from build123d import *

# Parameters (mm, degrees)
SKETCH2_R           = 19.05
BOSS_EXTRUDE1_DEPTH = 152.4
BOSS_EXTRUDE2_DEPTH = 12.7
SKETCH4_W           = 138.346275672
SKETCH4_H           = 79.731841005
BOSS_EXTRUDE3_DEPTH = 50.8
SKETCH5_W           = 63.5
SKETCH5_H           = 57.15
CUT_EXTRUDE1_DEPTH  = 132.116075905
CUT_EXTRUDE2_DEPTH  = 132.116075905
CUT_EXTRUDE3_DEPTH  = 124.514960069
SKETCH9_R           = 3.683
BOSS_EXTRUDE4_DEPTH = 25.4
CLEARANCECUT1_DEPTH = 109.569099969
CLEARANCECUT2_DEPTH = 12.954


with BuildPart() as part:
    # Sketch2 → Boss-Extrude1 (new body)
    with BuildSketch(Plane(origin=(0, 0, 0), x_dir=(1, 0, 0), z_dir=(0, 1, 0))):
        with Locations(Location((0, 0, 0), (0, 0, 90))):
            Circle(SKETCH2_R)
    extrude(amount=BOSS_EXTRUDE1_DEPTH)

    # Sketch3 → Boss-Extrude2 (add, symmetric)
    with BuildSketch(Plane.XY):
        Polygon((-427.750314484, -331.6732), (-409.789802242, -313.712687758), (-391.82929, -331.6732), align=None)
        Polygon((-6.028675512, 90.048438972), (-409.789802242, -313.712687758), (-391.82929, -331.6732), (11.93183673, 72.08792673), align=None)
    boss_extrude2 = extrude(amount=BOSS_EXTRUDE2_DEPTH, both=True)

    # Mirror1: Boss-Extrude2 across plane
    add(boss_extrude2.mirror(Plane(origin=(0, 0, 0), x_dir=(0, 0, 1), z_dir=(1, 0, 0))))


with BuildPart() as body_2:
    # Sketch4 → Boss-Extrude3 (new body)
    with BuildSketch(Plane.XY.offset(25.4)):
        with Locations((0, 59.259567455)):
            Rectangle(SKETCH4_W, SKETCH4_H)
    extrude(amount=-BOSS_EXTRUDE3_DEPTH)

    # Combine1: cut part
    add(part.part, mode=Mode.SUBTRACT)

    # Sketch5 → Cut-Extrude1 (cut, through all)
    with BuildSketch(Plane.XY.offset(25.4)):
        with Locations((0, 59.259567454)):
            Rectangle(SKETCH5_W, SKETCH5_H)
    extrude(amount=-CUT_EXTRUDE1_DEPTH, mode=Mode.SUBTRACT)

    # Sketch6 → Cut-Extrude2 (cut, through all)
    with BuildSketch(Plane.XY.offset(25.4)):
        Polygon((-69.173137836, 99.125487957), (-69.173137836, 44.864488891), (-40.730256121, 73.307370605), (-40.730256121, 99.125487957), align=None)
    cut_extrude2 = extrude(amount=-CUT_EXTRUDE2_DEPTH, mode=Mode.SUBTRACT)

    # Mirror2: Cut-Extrude2 across plane
    add(cut_extrude2.mirror(Plane(origin=(0, 0, 0), x_dir=(0, 0, 1), z_dir=(1, 0, 0))), mode=Mode.SUBTRACT)

    # Sketch8 → Cut-Extrude3 (cut, through all)
    with BuildSketch(Plane.XY):
        Polygon((69.173137836, 19.393646952), (69.173137836, 44.864488891), (40.730256121, 73.307370605), (40.730256121, 99.125487957), (-40.730256121, 99.125487957), (-40.730256121, 73.307370605), (-69.173137836, 44.864488891), (-69.173137836, 19.393646952), align=None)
    extrude(amount=-CUT_EXTRUDE3_DEPTH, mode=Mode.SUBTRACT)

    # Sketch9 → Boss-Extrude4 (add)
    with BuildSketch(Plane(origin=(0, 0, 0), x_dir=(-1, 0, 0), z_dir=(0, 0, -1))):
        with BuildLine():
            Line((-48.773997692, 65.263629035), (-39.369751391, 74.667875336))
            ThreePointArc((-39.369751391, 74.667875336), (-50.088798441, 81.199961636), (-52.36610014, 68.855731483))
            Line((-52.36610014, 68.855731483), (-48.773997692, 65.263629035))
        make_face()
        with Locations((-46.977946468, 74.243885156)):
            Circle(SKETCH9_R, mode=Mode.SUBTRACT)
    boss_extrude4 = extrude(amount=-BOSS_EXTRUDE4_DEPTH)

    # Mirror3: Boss-Extrude4 across plane
    add(boss_extrude4.mirror(Plane(origin=(0, 0, 0), x_dir=(0, 0, 1), z_dir=(1, 0, 0))))

    # Sketch10 → ClearanceCut1 (cut, through all)
    with BuildSketch(Plane.XZ.offset(-19.393646952)):
        with BuildLine():
            Line((-19.05, 0), (-19.304, 0))
            ThreePointArc((-19.304, 0), (0, 19.304), (19.304, 0))
            Line((19.304, 0), (19.05, 0))
            ThreePointArc((19.05, 0), (0, 19.05), (-19.05, 0))
        make_face()
    extrude(amount=-CLEARANCECUT1_DEPTH, mode=Mode.SUBTRACT)

    # Sketch11 → ClearanceCut2 (cut)
    with BuildSketch(Plane(origin=(0, 0, 0), x_dir=(-1, 0, 0), z_dir=(0, 0, -1))):
        Polygon((-69.173137836, 27.263186893), (-29.112312301, 67.324012428), (-29.112312301, 30.684567454), (-40.403232803, 19.393646952), (-69.173137836, 19.393646952), align=None)
    clearancecut2 = extrude(amount=-CLEARANCECUT2_DEPTH, mode=Mode.SUBTRACT)

    # Mirror4: ClearanceCut2 across plane
    add(clearancecut2.mirror(Plane(origin=(0, 0, 0), x_dir=(0, 0, 1), z_dir=(1, 0, 0))), mode=Mode.SUBTRACT)


solid = body_2.part
Build history of the part. All positions in model axes, mm. A direction names the side the tool comes from. Coordinates: 2 decimals unless noted, no trailing zeros. Order: outer loops, then holes, each group sorted by start corner. A loop starts at its lowest first (then second) coordinate and runs counter-clockwise, first axis right, second up. Notation, with made-up numbers: (-28.5, 7) - (-16.5, 7) arc R27 ccw to (-16.5, 42) - close; hole circle Ø11 at (70.25, 23). An arc over 180 degrees is marked (long way). Put each result on its own line as item: value.
1. Tool access for faces 4 (the face through (49, 32, 12.954)), 5 (the face through (59.12, 54.92, 12.88)), 6 (the face through (-59.12, 54.92, 12.88)), 7 (the face through (0, 30.685, 21)), 8 (the face through (69.173, 35, 13)): list every direction of +Z, -Z, +X, -X, +Y, -Y with a clear straight run to the whole face (end or side of a thin tool).
Answer sheet:
face 4: -Z
face 5: +Z, -Z, +X
face 6: +Z, -Z, -X
face 7: +Z, -Z
face 8: +Z, -Z, +X, +Y, -Y
2. Probe line 1 along X through (y, z) = (73, 11); line 2 along X through (y, z) = (71.5, 21.25); line 3 along Y through (x, z) = (3.5, 19.25). List the from-to ranges inside material, lowest first. Write a range as [from, to].
Answer sheet:
line 1: x = [-54.5, -50.44], [-43.51, -31.75], [31.75, 43.51], [50.44, 54.5]
line 2: x = [-54.09, -49.43], [-44.52, -31.75], [31.75, 44.52], [49.43, 54.09]
line 3: y = [19.39, 30.68], [87.83, 99.13]
3. Saw through at C-C (y = 53). Write the cut outline in (x, z).
Answer sheet:
outline: (-61.04, 0) - (-43.44, 0) - (-43.44, 12.95) - (-31.75, 12.95) - (-31.75, 25.4) - (-61.04, 25.4) - close; (31.75, 12.95) - (43.44, 12.95) - (43.44, 0) - (61.04, 0) - (61.04, 25.4) - (31.75, 25.4) - close
4. Saw through at D-D (x = 0). Write the cut outline in (y, z).
Answer sheet:
outline: (19.39, 19.3) - (30.68, 19.3) - (30.68, 25.4) - (19.39, 25.4) - close; (87.83, 19.3) - (99.13, 19.3) - (99.13, 25.4) - (87.83, 25.4) - close
5. Drop flat-ended pins along their axis: P1, Ø2, axis at x = 31, y = 32.5, coming from the -Z side; P2, Ø5, axis at y = 50, z = 21, coming from the -X side; P3, Ø2, axis at y = 54.5, z = 17, coming from the -X side. Give the stop position or say it passes through.
Answer sheet:
P1: stops at z = 12.95
P2: stops at x = -66.54
P3: stops at x = -60.54
6. Saw through at A-A (x = 27.5). Write the cut outline in (y, z), and give its area (3 significant figures).
Answer sheet:
outline: (19.39, 0) - (30.68, 0) - (30.68, 25.4) - (19.39, 25.4) - close; (87.83, 0) - (99.13, 0) - (99.13, 25.4) - (87.83, 25.4) - close
area: 574 mm^2
7. Saw through at B-B (z = 2). Give the number of separate pieces and of enclosed holes in the cut face, and give its area (3 significant figures).
Answer sheet:
separate pieces: 4
enclosed holes: 2
area: 2,570 mm^2
8. Pull direction Y, two halves, no side cores. Call faces 1 (the face through (-1, 99.125, 21)), 2 (the face through (27, 24, 0)), 3 (the face through (51.735, 80.196, 12.522)): pulls with the +Y half, pulls with the -Y half, needs draft (parallel to the pull), parting line crosses it, or undercut.
Answer sheet:
face 1: pulls with the +Y half
face 2: needs draft
face 3: undercut
